Verification items for the finished model (mm, model axes). A direction names the side the tool comes from. Round coordinates to 2 decimals unless told otherwise and drop trailing zeros. Write each loop counter-clockwise with the first axis right and the second up, starting at its lowest first coordinate (ties: lowest second). Pieces come first, ordered by that corner, then holes. Notation, with made-up numbers: M 8,79.25 L 56,79.25 A27 ccw 56,99.25 Z; hole C 25,-25.75 d3. An arc over 180 degrees is marked long. One line per item, written item: value. Start each with the question number.
Item 1: Thickness scan on probe 1 along Z at (x, y) = (-75.5, 0); probe 2 along Y at (x, z) = (74.5, 4); probe 3 along X at (y, z) = (3.5, 25). Record the ranges inside material, lowest first. Write a range as from..to.
Item 2: Section check C-C, the plane z = 29. Record the cut outline in (x, y).
Item 3: Gauge pin test, flat end, axial feed: pin 1 (9.5 mm diameter, centred on y = 1.5, z = 29.5, fed in from -X). Record the tip position at first contact, or that the pin passes through.
Item 4: Draft check along Y on faces 4 (the face through (-2, -32.5, 25)), 5 (the face through (-2, 0, 6)), 6 (the face through (-2, 32.5, 25)). Enter one of: +Y half, -Y half, draft (parallel to the pull), parting line (faces both ways), or undercut.
Item 5: Section check A-A, the plane x = -77. Record the cut outline in (y, z).
Item 6: Tool access check on faces 1 (the face through (-2, -3, 3)), 2 (the face through (-60.5, 0, 29)), 3 (the face through (-2, 18, 0)). Record the directions out of +Z, -Z, +X, -X, +Y, -Y that give a thin tool (end or side, any length) a straight path to the whole face; none if there is none.
Item 7: Section check B-B, the plane y = 0. Record the cut outline in (x, z), then the cut area to 3 significant figures.
from build123d import *

# Parameters (mm, degrees)
F0_W     = 225
F0_H     = 65
F1_DEPTH = 50
F2_R     = 9.5
F3_DEPTH = 52
F4_W     = 6
F4_H     = 6
F5_DEPTH = 325


with BuildPart() as f1:
    # F0 (on Top) → F1 (new body)
    with BuildSketch(Plane.XY):
        Rectangle(F0_W, F0_H)
    extrude(amount=F1_DEPTH)

    # F2 (on face) → F3 (cut)
    with BuildSketch(Plane(origin=(-112.5, 0, 0), x_dir=(0, -1, 0), z_dir=(-1, 0, 0))):
        with Locations((0, 29)):
            Circle(F2_R)
    extrude(amount=-F3_DEPTH, mode=Mode.SUBTRACT)

    # F4 (on face) → F5 (cut)
    with BuildSketch(Plane(origin=(-112.5, 0, 0), x_dir=(0, -1, 0), z_dir=(-1, 0, 0))):
        with Locations((0, 3)):
            Rectangle(F4_W, F4_H)
    extrude(amount=-F5_DEPTH, mode=Mode.SUBTRACT)


solid = f1.part
Response values:
1. probe 1: z = 6..19.5, 38.5..50
1. probe 2: y = -32.5..-3, 3..32.5
1. probe 3: x = -60.5..112.5
2. outline: M -112.5,-32.5 L 112.5,-32.5 L 112.5,32.5 L -112.5,32.5 L -112.5,9.5 L -60.5,9.5 L -60.5,-9.5 L -112.5,-9.5 Z
3. pin 1: stops at x = -60.5
4. face 4: -Y half
4. face 5: undercut
4. face 6: +Y half
5. outline: M -32.5,0 L -3,0 L -3,6 L 3,6 L 3,0 L 32.5,0 L 32.5,50 L -32.5,50 Z; hole C 0,29 d19
6. face 1: -Z, +X, -X
6. face 2: -X
6. face 3: -Z, +X, -X, +Y, -Y
7. outline: M -112.5,6 L 112.5,6 L 112.5,50 L -112.5,50 L -112.5,38.5 L -60.5,38.5 L -60.5,19.5 L -112.5,19.5 Z
7. area: 8,910 mm2
